Part print with two shaded views. Sizes in mm from the minimum x, y, z corner. Coordinates: 2 decimals unless noted, no trailing zeros. Loops run counter-clockwise (first coordinate to the right, second up) from the corner with the lowest first, then second, coordinate; pieces in that order, holes last.
Item 1: Flat gauge pin, fed straight in: pin 1 (7.5 mm diameter, centred on x = 15, z = 15, fed in from -Y). Where does the tip first touch, or does it go through?
Item 2: Cut at B-B (x = 15). List the corners of the cut face in (y, z).
Item 3: Cut at A-A (z = 135). List the corners of the cut face in (x, y), and give its area (3 significant figures).
Item 4: Drill centre lines: line 1 along Z through (x, y) = (15, 2.95); line 2 along X through (y, z) = (2.45, 15); line 3 along X through (y, z) = (3.8, 14). Where is each one in solid material? Low to high.
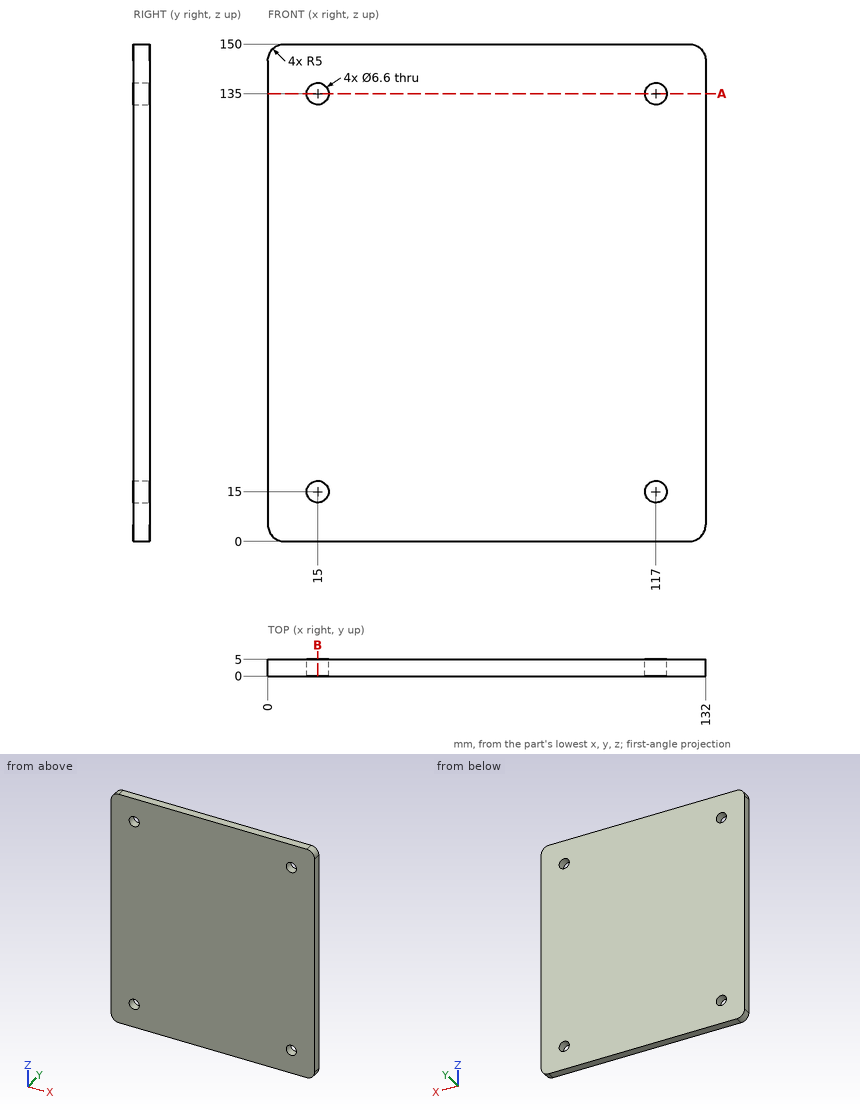
Filled sheet:
1. pin 1: stops at y = 0
2. outline: (0, 0) - (5, 0) - (5, 11.7) - (0, 11.7) - close; (0, 18.3) - (5, 18.3) - (5, 131.7) - (0, 131.7) - close; (0, 138.3) - (5, 138.3) - (5, 150) - (0, 150) - close
3. outline: (0, 0) - (11.7, 0) - (11.7, 5) - (0, 5) - close; (18.3, 0) - (113.7, 0) - (113.7, 5) - (18.3, 5) - close; (120.3, 0) - (132, 0) - (132, 5) - (120.3, 5) - close
3. area: 594 mm2
4. line 1: z = 0 to 11.7, 18.3 to 131.7, 138.3 to 150
4. line 2: x = 0 to 11.7, 18.3 to 113.7, 120.3 to 132
4. line 3: x = 0 to 11.86, 18.14 to 113.86, 120.14 to 132
